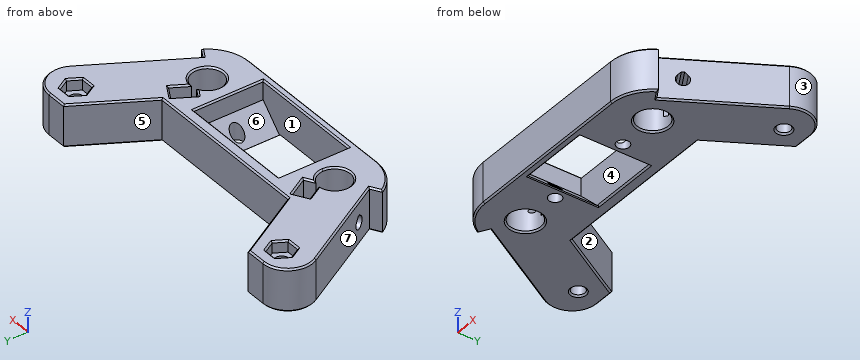
from build123d import *

# Parameters (mm, degrees)
SKETCH1_R           = 4.05
SKETCH1_R_2         = 1.7
SKETCH1_W           = 18
SKETCH1_H           = 18
BOSS_EXTRUDE1_DEPTH = 11
SKETCH11_W          = 30
SKETCH11_H          = 18
CUT_EXTRUDE9_DEPTH  = 5
CUT_EXTRUDE4_DEPTH  = 16
CUT_EXTRUDE5_START  = -10
CUT_EXTRUDE5_DEPTH  = 4
CUT_EXTRUDE7_DEPTH  = 57.773728613
CUT_EXTRUDE8_DEPTH  = 3
CHAMFER1_SIZE       = 0.4
CHAMFER2_SIZE       = 0.4
CHAMFER3_SIZE       = 6
SKETCH12_R          = 1.65
CUT_EXTRUDE10_DEPTH = 55.621156131


with BuildPart() as part:
    # Sketch1 → Boss-Extrude1 (new body)
    with BuildSketch(Plane.XY):
        with BuildLine():
            Line((-29.42820323, -4), (-46.92820323, 26.310889132))
            Line((-46.92820323, 26.310889132), (-40.538475773, 30))
            Line((-40.538475773, 30), (-32.661364738, 30))
            Line((-32.661364738, 30), (-22.269059892, 12))
            Line((-22.269059892, 12), (22.269059892, 12))
            Line((22.269059892, 12), (32.661364738, 30))
            Line((32.661364738, 30), (40.538475773, 30))
            Line((40.538475773, 30), (46.92820323, 26.310889132))
            Line((46.92820323, 26.310889132), (29.42820323, -4))
            Line((29.42820323, -4), (32.026279442, -5.5))
            ThreePointArc((32.026279442, -5.5), (28, -9.526279442), (22.5, -11))
            Line((22.5, -11), (-22.5, -11))
            ThreePointArc((-22.5, -11), (-28, -9.526279442), (-32.026279442, -5.5))
            Line((-32.026279442, -5.5), (-29.42820323, -4))
        make_face()
        with Locations((-22.5, 0)):
            Circle(SKETCH1_R, mode=Mode.SUBTRACT)
        with Locations(Location((22.5, 0, 0), (0, 0, 180))):
            Circle(SKETCH1_R, mode=Mode.SUBTRACT)
        with Locations((-36.356406461, 24)):
            Circle(SKETCH1_R_2, mode=Mode.SUBTRACT)
        with Locations((36.356406461, 24)):
            Circle(SKETCH1_R_2, mode=Mode.SUBTRACT)
        Rectangle(SKETCH1_W, SKETCH1_H, mode=Mode.SUBTRACT)
    extrude(amount=BOSS_EXTRUDE1_DEPTH)

    # Sketch11 → Cut-Extrude9 (cut)
    with BuildSketch(Plane.XY.offset(11)):
        Rectangle(SKETCH11_W, SKETCH11_H)
    extrude(amount=-CUT_EXTRUDE9_DEPTH, mode=Mode.SUBTRACT)

    # Sketch6 → Cut-Extrude4 (cut)
    with BuildSketch(Plane(origin=(-23.80320323, -13.742785793, 0), x_dir=(0, 0, 1), z_dir=(-0.8660254037844398, -0.4999999999999983, 0))):
        with BuildLine():
            Line((6.63137085, 15.61862915), (7.42, 16.4072583))
            Line((7.42, 16.4072583), (7.42, 17.0927417))
            Line((7.42, 17.0927417), (6.63137085, 17.88137085))
            ThreePointArc((6.63137085, 17.88137085), (3.9, 16.75), (6.63137085, 15.61862915))
        make_face()
    cut_extrude4 = extrude(amount=-CUT_EXTRUDE4_DEPTH, mode=Mode.SUBTRACT)

    # Sketch7 → Cut-Extrude5 (cut)
    with BuildSketch(Plane(origin=(-23.80320323, -13.742785793, 0), x_dir=(0, 0, 1), z_dir=(-0.8660254037844398, -0.4999999999999983, 0)).offset(CUT_EXTRUDE5_START)):
        Polygon((11, 19.65), (11, 13.85), (3.625684219, 13.85), (1.951368439, 16.75), (3.625684219, 19.65), align=None)
    cut_extrude5 = extrude(amount=-CUT_EXTRUDE5_DEPTH, mode=Mode.SUBTRACT)

    # Mirror2: Cut-Extrude4, Cut-Extrude5 across plane
    add(cut_extrude4.mirror(Plane(origin=(0, 0, 0), x_dir=(0, 0, 1), z_dir=(1, 0, 0))), mode=Mode.SUBTRACT)
    add(cut_extrude5.mirror(Plane(origin=(0, 0, 0), x_dir=(0, 0, 1), z_dir=(1, 0, 0))), mode=Mode.SUBTRACT)

    # Sketch9 → Cut-Extrude7 (cut, through all)
    with BuildSketch(Plane.XY.offset(11)):
        with BuildLine():
            Line((-43.428947258, 20.25), (-46.92820323, 26.310889132))
            Line((-46.92820323, 26.310889132), (-40.538475773, 30))
            Line((-40.538475773, 30), (-37.799782134, 30))
            ThreePointArc((-37.799782134, 30), (-43.428947258, 26.75), (-43.428947258, 20.25))
        make_face()
        with BuildLine():
            Line((40.538475773, 30), (37.799782134, 30))
            ThreePointArc((37.799782134, 30), (43.428947258, 26.75), (43.428947258, 20.25))
            Line((43.428947258, 20.25), (46.92820323, 26.310889132))
            Line((46.92820323, 26.310889132), (40.538475773, 30))
        make_face()
    extrude(amount=-CUT_EXTRUDE7_DEPTH, mode=Mode.SUBTRACT)

    # Sketch10 → Cut-Extrude8 (cut)
    with BuildSketch(Plane.XY.offset(11)):
        Polygon((39.705038022, 24), (38.030722241, 26.9), (34.68209068, 26.9), (33.007774899, 24), (34.68209068, 21.1), (38.030722241, 21.1), align=None)
        Polygon((-33.007774899, 24), (-34.68209068, 26.9), (-38.030722241, 26.9), (-39.705038022, 24), (-38.030722241, 21.1), (-34.68209068, 21.1), align=None)
    extrude(amount=-CUT_EXTRUDE8_DEPTH, mode=Mode.SUBTRACT)

    # Chamfer1
    chamfer1_edges = [part.edges().sort_by_distance(p)[0] for p in [
        (0, -11, 11),
        (-25.353578994, -2.873949708, 11),
        (-23.748378775, 6.162255466, 11),
        (-20.053847577, 7.763139721, 11),
        (-23.235898385, 9.274613392, 11),
        (-19.857316504, 4.527975428, 11),
        (28, -9.526279442, 11),
        (30.727241336, -4.75, 11),
        (25.353578994, -2.873949708, 11),
        (23.235898385, 9.274613392, 11),
        (19.857316504, 4.527975428, 11),
        (23.748378775, 6.162255466, 11),
        (20.053847577, 7.763139721, 11),
        (36.428575244, 8.125, 11),
        (-36.428575244, 8.125, 11),
        (-43.428947258, 26.75, 11),
        (35.230573436, 30, 11),
        (43.428947258, 26.75, 11),
        (38.867880132, 22.55, 11),
        (38.867880132, 25.45, 11),
        (36.356406461, 26.9, 11),
        (33.84493279, 25.45, 11),
        (33.84493279, 22.55, 11),
        (36.356406461, 21.1, 11),
        (-33.84493279, 22.55, 11),
        (-33.84493279, 25.45, 11),
        (-36.356406461, 26.9, 11),
        (-38.867880132, 25.45, 11),
        (-38.867880132, 22.55, 11),
        (-36.356406461, 21.1, 11),
        (27.465212315, 21, 11),
        (0, 12, 11),
        (-27.465212315, 21, 11),
        (-35.230573436, 30, 11),
        (-30.727241336, -4.75, 11),
        (0, -9, 11),
        (0, 9, 11),
        (-28, -9.526279442, 11),
        (-15, 0, 11),
        (15, 0, 11),
    ]]
    chamfer(chamfer1_edges, length=CHAMFER1_SIZE)

    # Chamfer2
    chamfer2_edges = [part.edges().sort_by_distance(p)[0] for p in [
        (-35.230573436, 30, 0),
        (-27.465212315, 21, 0),
        (0, 12, 0),
        (27.465212315, 21, 0),
        (36.428575244, 8.125, 0),
        (30.727241336, -4.75, 0),
        (28, -9.526279442, 0),
        (0, -11, 0),
        (-28, -9.526279442, 0),
        (-30.727241336, -4.75, 0),
        (-36.428575244, 8.125, 0),
        (-43.428947258, 26.75, 0),
        (35.230573436, 30, 0),
        (43.428947258, 26.75, 0),
        (-26.55, 0, 0),
        (26.55, 0, 0),
        (-9, 0, 0),
        (0, -9, 0),
        (9, 0, 0),
        (0, 9, 0),
        (-38.056406461, 24, 0),
        (34.656406461, 24, 0),
    ]]
    chamfer(chamfer2_edges, length=CHAMFER2_SIZE)

    # Chamfer3
    # the kernel refuses this chamfer: 6 mm, written as the material it takes off along each edge
    with BuildSketch(Plane(origin=(-9, -9, 6), x_dir=(0.02749587661058649, 0, -0.9996219169112968), z_dir=(0, 1, 0)), Plane(origin=(9, 9, 6), x_dir=(-0.02749587661058649, 0, -0.9996219169112968), z_dir=(0, -1, 0))) as chamfer3_piece_1:
        Polygon((CHAMFER3_SIZE * 0.999621916911, CHAMFER3_SIZE * 0.0274958766106), (-CHAMFER3_SIZE * 0.0274958766106, CHAMFER3_SIZE * 0.999621916911), (0, 0), align=None)
    extrude(amount=18, mode=Mode.SUBTRACT)

    # Sketch12 → Cut-Extrude10 (cut, through all)
    with BuildSketch(Plane(origin=(0, 0, 0), x_dir=(-1, 0, 0), z_dir=(0, 0, -1))):
        with Locations((12, 0)):
            Circle(SKETCH12_R)
        with Locations((-12, 0)):
            Circle(SKETCH12_R)
    extrude(amount=-CUT_EXTRUDE10_DEPTH, mode=Mode.SUBTRACT)


solid = part.part
Could you check a few things on this model? Use its own coordinates, in mm. Face numbers are marked on the shaded views. A direction names the side the tool comes from. Give positions to 0.01 mm unless a question says otherwise; leave off trailing zeros. Order: outer loops, then holes, each group sorted by start corner. A loop starts at its lowest first (then second) coordinate and runs counter-clockwise, first axis right, second up. Notation, with made-up numbers: (23, -19) -> (28, -19) arc R16 cw to (28, -8) -> close; hole circle Ø4 at (51.5, -33). An arc over 180 degrees is marked (long way). Answer in a Markdown table with one row per item. Add a question column.
Item 1: I'm going to push flat-ended pins straight in: P1, Ø6.5, axis at x = 34.5, y = 24.5, coming from the +Z side; P2, Ø2, axis at x = 36, z = 9, coming from the -Y side; P3, Ø1.3, axis at x = -36, z = 9, coming from the -Y side; P4, Ø2.5, axis at y = -3.5, z = 9, coming from the +X side. Where does each tip first touch, or does it pass through?
Item 2: Please list where these lines run through material, in increasing order: probe 1 along X at (y, z) = (0, 1.4); probe 2 along X at (y, z) = (1.5, 6.75); probe 3 along Y at (x, z) = (12, 2.45).
Item 3: Imagine slicing it at C-C (z = 9.75). Count the separate pieces of the cut face and the enclosed holes in it, and give its area (3 significant figures).
Item 4: Imagine slicing it at B-B (y = 19). List the corners of the cut face in (x, z) for me, and give its area (3 significant figures).
Item 5: We'd pull the mould along Y, two halves only. Please class the marked faces 1, 2, 3 and 4: pulls with the +Y half, pulls with the -Y half, needs draft (parallel to the pull), parting line crosses it, or undercut.
Item 6: Imagine slicing it at A-A (x = 12). List the corners of the cut face in (y, z) for me.
Item 7: For the marked faces 5, 6 and 7, which set-ups out of +Z, -Z, +X, -X, +Y, -Y let a thin tool reach every point of the face, with its end or its side?
Result:
| question | item | result |
|---|---|---|
| 1 | P1 | z = 11 |
| 1 | P2 | y = 5.65 |
| 1 | P3 | y = 6.26 |
| 1 | P4 | x = 30.73 |
| 2 | probe 1 | -31.74 to -26.55, -18.45 to -13.65, 13.65 to 18.45, 26.55 to 31.74 |
| 2 | probe 2 | -28.88 to -26.26, -18.74 to -15, 15 to 18.74, 26.26 to 28.88 |
| 2 | probe 3 | -11 to -1.65, 1.65 to 12 |
| 3 | separate pieces | 1 |
| 3 | enclosed holes | 5 |
| 3 | area | 1,290 mm2 |
| 4 | outline | (-42.71, 0.4) -> (-42.25, 0) -> (-26.77, 0) -> (-26.31, 0.4) -> (-26.31, 10.6) -> (-26.77, 11) -> (-42.25, 11) -> (-42.71, 10.6) -> close; (26.31, 0.4) -> (26.77, 0) -> (42.25, 0) -> (42.71, 0.4) -> (42.71, 10.6) -> (42.25, 11) -> (26.77, 11) -> (26.31, 10.6) -> close |
| 4 | area | 360 mm2 |
| 5 | face 1 | undercut |
| 5 | face 2 | pulls with the +Y half |
| 5 | face 3 | parting line crosses it |
| 5 | face 4 | undercut |
| 6 | outline | (-11, 0.4) -> (-10.6, 0) -> (-1.65, 0) -> (-1.65, 3) -> (-9, 3) -> (-9, 10.6) -> (-9.4, 11) -> (-10.6, 11) -> (-11, 10.6) -> close; (1.65, 0) -> (11.6, 0) -> (12, 0.4) -> (12, 10.6) -> (11.6, 11) -> (9.4, 11) -> (9, 10.6) -> (9, 3) -> (1.65, 3) -> close |
| 7 | face 5 | +Z, -Z, +Y |
| 7 | face 6 | +Z |
| 7 | face 7 | +Z, -Z, -X |
